from build123d import *

# Parameters (mm, degrees)
BOSS_EXTRUDE1_DEPTH     = 3
SKETCH2_R               = 7.546344396
SKETCH2_R_2             = 6.998827146
SKETCH2_W               = 3
SKETCH2_H               = 30
SKETCH2_H_2             = 7
CUT_EXTRUDE1_DEPTH      = 1
CUT_EXTRUDE1_DEPTH_BACK = 4


with BuildPart() as part:
    # Sketch1 → Boss-Extrude1 (new body)
    with BuildSketch(Plane.XY):
        with BuildLine():
            Line((-11.521707287, -45.747254375), (11.521707287, -45.747254375))
            ThreePointArc((11.521707287, -45.747254375), (24.576520143, -40.046827338), (30, -26.874550642))
            Line((30, -26.874550642), (30, 7.734550642))
            ThreePointArc((30, 7.734550642), (24.576520143, 20.906827338), (11.521707287, 26.607254375))
            Line((11.521707287, 26.607254375), (-11.521707287, 26.607254375))
            ThreePointArc((-11.521707287, 26.607254375), (-24.576520143, 20.906827338), (-30, 7.734550642))
            Line((-30, 7.734550642), (-30, -26.874550642))
            ThreePointArc((-30, -26.874550642), (-24.576520143, -40.046827338), (-11.521707287, -45.747254375))
        make_face()
    extrude(amount=BOSS_EXTRUDE1_DEPTH)

    # Sketch2 → Cut-Extrude1 (cut, two sides)
    with BuildSketch(Plane.XY.offset(3)) as cut_extrude1_sk:
        with Locations((-20.712852781, -10.370577489)):
            Circle(SKETCH2_R)
        with Locations((-20.641158555, -26.754776444)):
            Circle(SKETCH2_R_2)
        with Locations((20.641158555, -26.754776444)):
            Circle(SKETCH2_R_2)
        with Locations((20.712852781, -10.370577489)):
            Circle(SKETCH2_R)
        with Locations((-9.5, -20.747254375)):
            Rectangle(SKETCH2_W, SKETCH2_H)
        with Locations((9.5, -20.747254375)):
            Rectangle(SKETCH2_W, SKETCH2_H)
        with BuildLine():
            Line((-12.367254006, 18.139818395), (12.367254006, 18.139818395))
            ThreePointArc((12.367254006, 18.139818395), (19.070664148, 11.436408253), (12.367254006, 4.732998111))
            Line((12.367254006, 4.732998111), (-12.367254006, 4.732998111))
            ThreePointArc((-12.367254006, 4.732998111), (-19.070664148, 11.436408253), (-12.367254006, 18.139818395))
        make_face()
        with BuildLine():
            Line((5.484608298, -9.027083299), (5.484608298, -38.747254375))
            ThreePointArc((5.484608298, -38.747254375), (0, -44.231862673), (-5.484608298, -38.747254375))
            Line((-5.484608298, -38.747254375), (-5.484608298, -9.027083299))
            ThreePointArc((-5.484608298, -9.027083299), (0, -3.542475001), (5.484608298, -9.027083299))
        make_face()
        with Locations((10.5, -42.247254375)):
            Rectangle(SKETCH2_W, SKETCH2_H_2)
        with Locations((-10.5, -42.247254375)):
            Rectangle(SKETCH2_W, SKETCH2_H_2)
        with Locations((-10.5, 23.107254375)):
            Rectangle(SKETCH2_W, SKETCH2_H_2)
        with Locations((10.5, 23.107254375)):
            Rectangle(SKETCH2_W, SKETCH2_H_2)
    extrude(amount=CUT_EXTRUDE1_DEPTH, mode=Mode.SUBTRACT)
    extrude(cut_extrude1_sk.sketch, amount=-CUT_EXTRUDE1_DEPTH_BACK, mode=Mode.SUBTRACT)


solid = part.part
Build history of the part. All positions in model axes, mm. A direction names the side the tool comes from. Round coordinates to 2 decimals unless told otherwise and drop trailing zeros. Write each loop counter-clockwise with the first axis right and the second up, starting at its lowest first coordinate (ties: lowest second). Pieces come first, ordered by that corner, then holes. Notation, with made-up numbers: (13, -8) -> (52, -8) arc R25 cw to (52, 19) -> close; hole circle Ø6 at (55, 59). An arc over 180 degrees is marked (long way). Use one line per item in the form item = value.
Q1. Drop flat-ended pins along their axis: P1, Ø0.9, axis at x = -10, z = 1, coming from the +Y side; P2, Ø1.5, axis at y = 21.5, z = 1, coming from the +X side; P3, Ø0.9, axis at x = -10, z = 1.5, coming from the -Y side. Give the stop position or say it passes through.
Conclusion:
P1 = 19.61
P2 = 24.73
P3 = -38.75
Q2. Band-saw the part on C-C, the plane y = -14. Write the cut outline in (x, z).
Conclusion:
outline = (-30, 0) -> (-27.33, 0) -> (-27.33, 3) -> (-30, 3) -> close; (-14.1, 0) -> (-11, 0) -> (-11, 3) -> (-14.1, 3) -> close; (-8, 0) -> (-5.48, 0) -> (-5.48, 3) -> (-8, 3) -> close; (5.48, 0) -> (8, 0) -> (8, 3) -> (5.48, 3) -> close; (11, 0) -> (14.1, 0) -> (14.1, 3) -> (11, 3) -> close; (27.33, 0) -> (30, 0) -> (30, 3) -> (27.33, 3) -> close
Q3. Band-saw the part on D-D, the plane x = -17. Write the cut outline in (y, z).
Conclusion:
outline = (-44.78, 0) -> (-32.73, 0) -> (-32.73, 3) -> (-44.78, 3) -> close; (-20.78, 0) -> (-16.94, 0) -> (-16.94, 3) -> (-20.78, 3) -> close; (-3.8, 0) -> (6.59, 0) -> (6.59, 3) -> (-3.8, 3) -> close; (16.28, 0) -> (25.64, 0) -> (25.64, 3) -> (16.28, 3) -> close
Q4. Drill centre lines: L1, parallel to X at y = -18.5, z = 0.85; L2, parallel to Y at x = -10.5, z = 1.45; L3, parallel to Y at x = 0, z = 1.15. Where is each one in solid material? Low to high.
Conclusion:
L1 = -30 to -11, -8 to -5.48, 5.48 to 8, 11 to 30
L2 = -38.75 to -35.75, -5.75 to 4.73, 18.14 to 19.61
L3 = -45.75 to -44.23, -3.54 to 4.73, 18.14 to 26.61
Q5. Tool access for faces 4 (the cylindrical face through (-24.6, 20.88, 1.48)), 5 (the flat face through (-11, 19.607, 2)), 6 (the flat face through (-12, -42, 2)), 7 (the flat face through (-10, -35.747, 2)), 8 (the flat face through (-30, -9, 1)): list every direction of +Z, -Z, +X, -X, +Y, -Y with a clear straight run to the whole face (end or side of a thin tool).
Conclusion:
face_4 = +Z, -Z, -X, +Y
face_5 = +Z, -Z, +Y
face_6 = +Z, -Z, -Y
face_7 = +Z, -Z
face_8 = +Z, -Z, -X, +Y, -Y
Q6. Two-plate mould, pull along Y, no slides. Class faces 1 (the flat face through (-12, 23, 2)), 2 (the cylindrical face through (24.88, 20.59, 1.48)), 3 (the cylindrical face through (-13.966, -24.653, 1.521)): released by +Y, released by -Y, zero draft, split by the parting line, or undercut.
Conclusion:
face_1 = zero draft
face_2 = released by +Y
face_3 = undercut
Q7. Band-saw the part on A-A, the plane y = 13.5. Write the cut outline in (x, z).
Conclusion:
outline = (-29.07, 0) -> (-18.75, 0) -> (-18.75, 3) -> (-29.07, 3) -> close; (18.75, 0) -> (29.07, 0) -> (29.07, 3) -> (18.75, 3) -> close
Q8. Band-saw the part on B-B, the plane x = 0. Write the cut outline in (y, z), then the cut area to 3 significant figures.
Conclusion:
outline = (-45.75, 0) -> (-44.23, 0) -> (-44.23, 3) -> (-45.75, 3) -> close; (-3.54, 0) -> (4.73, 0) -> (4.73, 3) -> (-3.54, 3) -> close; (18.14, 0) -> (26.61, 0) -> (26.61, 3) -> (18.14, 3) -> close
area = 54.8 mm²
